The listing builds one solid part. Answer for the finished solid, in the listing's coordinates (mm). Face numbers are marked on the shaded views. Coordinates: 2 decimals unless noted, no trailing zeros. Write each loop counter-clockwise with the first axis right and the second up, starting at its lowest first coordinate (ties: lowest second). Pieces come first, ordered by that corner, then holes.
(1) The part is cut by section C-C on x = 2.35. Determine the outline of the cut face in (y, z).
(2) The part is cut by section D-D on z = -5.75. Determine the outline of the cut face in (x, y).
(3) Straight lines are drawn through the part: line 1 (Y direction, x = 1.35, z = -4); line 2 (Z direction, x = 1.4, y = 5.5); line 3 (Y direction, x = 1, z = -13.5). For each, find the intervals that lie inside material, in ascending order.
(4) For a pull along Y with two mould halves and no side action, classify the marked faces 1, 2 and 3 as +Y half, -Y half, draft (parallel to the pull), parting line (faces both ways), or undercut.
(5) The part is cut by section A-A on y = 5. Give the number of separate pieces and of enclosed holes in the cut face, plus the area to 3 significant figures.
(6) The part is cut by section B-B on z = -14. Determine the outline of the cut face in (x, y).
Autodesk Inventor part; units mm, degrees
ref_plane "YZ Plane" through (0, 0, 0) normal (1, 0, 0) x (0, 1, 0)
ref_plane "XZ Plane" through (0, 0, 0) normal (0, 1, 0) x (-1, 0, 0)
ref_plane "XY Plane" through (0, 0, 0) normal (0, 0, 1) x (1, 0, 0)
sketch "Sketch1" plane through (0, 0, 0) normal (1, 0, 0) x (0, 1, 0)
  point P0 (0, 0)
sketch "Sketch2" plane through (0, 0, 0) normal (1, 0, 0) x (0, 1, 0)
  line L0 (0, 0) -> (10, 0)
  line L1 (10, 0) -> (10, -20)
  line L2 (10, -20) -> (0, -20)
  line L3 (0, -20) -> (0, 0)
  dimension "d0" = 10
  dimension "d1" = 20
extrude "Extrusion1" add sketch "Sketch2" along normal blind 3
fillet "Fillet1" radius 3 1 edges at (1.5, 10, 0)
fillet "Fillet2" radius 3 1 edges at (1.5, 0, 0)
fillet "Fillet3" radius 3 1 edges at (3, 5, -20)
sketch "Sketch3" plane through (3, 0, 0) normal (1, 0, 0) x (0, 0, -1)
  circle A0 centre (4, 5) radius 2
  point P0 (0, 0)
  dimension "d14" = 4
extrude "Extrusion2" cut sketch "Sketch3" against normal blind 3
sketch "Sketch4" plane through (3, 0, 0) normal (1, 0, 0) x (0, 0, -1)
  circle A0 centre (14, 5) radius 2
  point P0 (0, 0)
  dimension "d10" = 4
extrude "Extrusion3" cut sketch "Sketch4" against normal blind 3
properties part number "holder 1"
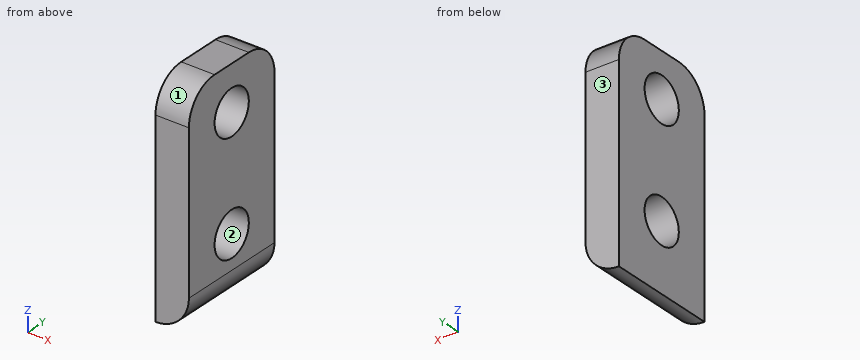
Model answer:
1. outline: (0, -18.87) - (10, -18.87) - (10, -3) arc R3 ccw to (7, 0) - (3, 0) arc R3 ccw to (0, -3) - close; hole circle Ø4 at (5, -14); hole circle Ø4 at (5, -4)
2. outline: (0, 0) - (3, 0) - (3, 4.03) - (0, 4.03) - close; (0, 5.97) - (3, 5.97) - (3, 10) - (0, 10) - close
3. line 1: y = 0 to 3, 7 to 10
3. line 2: z = -19.65 to -15.94, -12.06 to -5.94, -2.06 to 0
3. line 3: y = 0 to 3.06, 6.94 to 10
4. face 1: -Y half
4. face 2: undercut
4. face 3: +Y half
5. separate pieces: 3
5. enclosed holes: 0
5. area: 34.1 mm2
6. outline: (0, 0) - (3, 0) - (3, 3) - (0, 3) - close; (0, 7) - (3, 7) - (3, 10) - (0, 10) - close
